Check sheet for the modelled part. Datum: model origin and axes. Units: mm. Round coordinates to 2 decimals unless told otherwise and drop trailing zeros. Write each loop counter-clockwise with the first axis right and the second up, starting at its lowest first coordinate (ties: lowest second). Pieces come first, ordered by that corner, then holes.
Item 1: Section check D-D, the plane y = 1.8. State how many separate pieces and enclosed holes the cut face has, plus the area to 3 significant figures.
Item 2: Material ranges on line 1 along X through (y, z) = (2.55, 39); line 2 along X through (y, z) = (0.75, 24.5); line 3 along X through (y, z) = (2.2, 43.5), recorded low to high.
Item 3: Section check A-A, the plane z = 49. Record the cut outline in (x, y).
Item 4: Section check C-C, the plane x = 16.25. Record the cut outline in (y, z), plus the area to 3 significant figures.
Item 5: Depth check by flat-ended pin: pin 1 (3.5 mm diameter, centred on x = -42.44, z = -24.5, fed in from -Y). Enter the tip coordinate at first touch or a pass-through.
Item 6: Section check B-B, the plane z = -36. Record the cut outline in (x, y), plus the area to 3 significant figures.
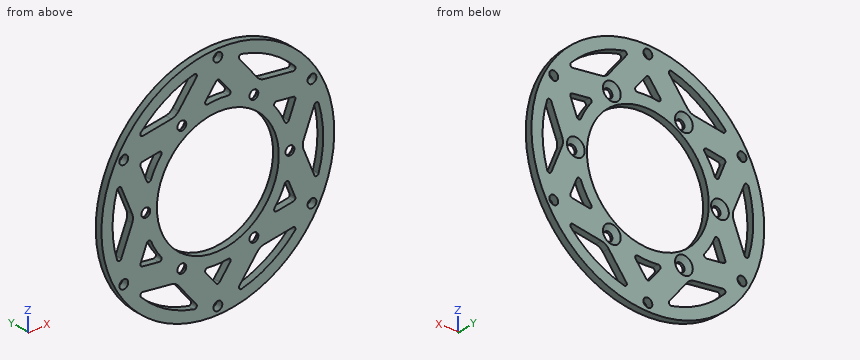
from build123d import *

# Parameters (mm, degrees)
SKETCH_1_R               = 52.5
SKETCH_1_R_2             = 2
SKETCH_1_R_3             = 27.5
EXTRUDE_1_DEPTH          = 3
HOLE_WIZARD_1_AT_2_COUNT = 2
HOLE_WIZARD_1_AT_2_PITCH = 32.5
HOLE_WIZARD_1_AT_3_COUNT = 2
HOLE_WIZARD_1_AT_3_PITCH = 56.291651246
HOLE_WIZARD_1_AT_4_COUNT = 2
HOLE_WIZARD_1_AT_4_PITCH = 65
HOLE_WIZARD_1_AT_5_COUNT = 2
HOLE_WIZARD_1_AT_5_PITCH = 56.291651246
HOLE_WIZARD_1_AT_6_COUNT = 2
HOLE_WIZARD_1_AT_6_PITCH = 32.5
CUT_EXTRUDE_1_DEPTH      = 10
FILLET_1_R               = 5
FILLET_2_R               = 1


with BuildPart() as part:
    # 草图1 → 凸台-拉伸1 (new body)
    with BuildSketch(Plane(origin=(0, 0, 0), x_dir=(1, 0, 0), z_dir=(0, 1, 0))):
        with Locations(Location((0, 0, 0), (0, 0, 270))):
            Circle(SKETCH_1_R)
        with Locations(Location((0, 49, 0), (0, 0, 270))):
            Circle(SKETCH_1_R_2, mode=Mode.SUBTRACT)
        with Locations(Location((-16.25, 28.145825623, 0), (0, 0, 270))):
            Circle(SKETCH_1_R_2, mode=Mode.SUBTRACT)
        with Locations(Location((42.435244785, 24.5, 0), (0, 0, 270))):
            Circle(SKETCH_1_R_2, mode=Mode.SUBTRACT)
        with Locations(Location((16.25, 28.145825623, 0), (0, 0, 270))):
            Circle(SKETCH_1_R_2, mode=Mode.SUBTRACT)
        with Locations(Location((42.435244785, -24.5, 0), (0, 0, 270))):
            Circle(SKETCH_1_R_2, mode=Mode.SUBTRACT)
        with Locations(Location((32.5, 0, 0), (0, 0, 270))):
            Circle(SKETCH_1_R_2, mode=Mode.SUBTRACT)
        with Locations(Location((0, -49, 0), (0, 0, 270))):
            Circle(SKETCH_1_R_2, mode=Mode.SUBTRACT)
        with Locations(Location((16.25, -28.145825623, 0), (0, 0, 270))):
            Circle(SKETCH_1_R_2, mode=Mode.SUBTRACT)
        with Locations(Location((-42.435244785, -24.5, 0), (0, 0, 270))):
            Circle(SKETCH_1_R_2, mode=Mode.SUBTRACT)
        with Locations(Location((-16.25, -28.145825623, 0), (0, 0, 270))):
            Circle(SKETCH_1_R_2, mode=Mode.SUBTRACT)
        with Locations(Location((-42.435244785, 24.5, 0), (0, 0, 270))):
            Circle(SKETCH_1_R_2, mode=Mode.SUBTRACT)
        with Locations(Location((-32.5, 0, 0), (0, 0, 270))):
            Circle(SKETCH_1_R_2, mode=Mode.SUBTRACT)
        with Locations(Location((0, 0, 0), (0, 0, 270))):
            Circle(SKETCH_1_R_3, mode=Mode.SUBTRACT)
    extrude(amount=EXTRUDE_1_DEPTH)

    # 草图3 → 孔1 (revolve, cut)
    with BuildSketch(Plane(origin=(-16.25, 3, -28.145825623), x_dir=(0, 0, 1), z_dir=(1, 0, 0))):
        Polygon((0, 0), (0, 3), (2, 3), (2, 2), (4, 0), align=None)
    hole_wizard_1 = revolve(axis=Axis((-16.25, 9.445314094, -28.145825623), (0, -1, 0)), mode=Mode.SUBTRACT)

    # 孔1 at 2: 孔1 ×2
    with Locations(*[(i * HOLE_WIZARD_1_AT_2_PITCH, 0, 0) for i in range(1, HOLE_WIZARD_1_AT_2_COUNT)]):
        add(hole_wizard_1, mode=Mode.SUBTRACT)

    # 孔1 at 3: 孔1 ×2
    with Locations(*[Vector(0.8660254037844387, 0, 0.5) * (i * HOLE_WIZARD_1_AT_3_PITCH) for i in range(1, HOLE_WIZARD_1_AT_3_COUNT)]):
        add(hole_wizard_1, mode=Mode.SUBTRACT)

    # 孔1 at 4: 孔1 ×2
    with Locations(*[Vector(0.5000000000000001, 0, 0.8660254037844386) * (i * HOLE_WIZARD_1_AT_4_PITCH) for i in range(1, HOLE_WIZARD_1_AT_4_COUNT)]):
        add(hole_wizard_1, mode=Mode.SUBTRACT)

    # 孔1 at 5: 孔1 ×2
    with Locations(*[(0, 0, i * HOLE_WIZARD_1_AT_5_PITCH) for i in range(1, HOLE_WIZARD_1_AT_5_COUNT)]):
        add(hole_wizard_1, mode=Mode.SUBTRACT)

    # 孔1 at 6: 孔1 ×2
    with Locations(*[Vector(-0.5000000000000003, 0, 0.8660254037844386) * (i * HOLE_WIZARD_1_AT_6_PITCH) for i in range(1, HOLE_WIZARD_1_AT_6_COUNT)]):
        add(hole_wizard_1, mode=Mode.SUBTRACT)

    # 草图5 → 切除-拉伸1 (cut)
    with BuildSketch(Plane(origin=(0, 3, 0), x_dir=(1, 0, 0), z_dir=(0, 1, 0))):
        with BuildLine():
            Line((-8.041886602, 46.814293329), (-18.947738206, 32.818445262))
            Line((-18.947738206, 32.818445262), (-36.521423982, 30.371624756))
            ThreePointArc((-36.521423982, 30.371624756), (-23.75, 41.13620668), (-8.041886602, 46.814293329))
        make_face()
        with BuildLine():
            Line((0, 40.865281716), (7.136483547, 31.706791111))
            ThreePointArc((7.136483547, 31.706791111), (0, 32.5), (-7.136483547, 31.706791111))
            Line((-7.136483547, 31.706791111), (0, 40.865281716))
        make_face()
        with BuildLine():
            Line((18.947738206, 32.818445262), (8.041886602, 46.814293329))
            ThreePointArc((8.041886602, 46.814293329), (23.75, 41.13620668), (36.521423982, 30.371624756))
            Line((36.521423982, 30.371624756), (18.947738206, 32.818445262))
        make_face()
        with BuildLine():
            Line((35.390372099, 20.432640858), (23.890644801, 22.033771601))
            ThreePointArc((23.890644801, 22.033771601), (28.145825623, 16.25), (31.027128348, 9.67301951))
            Line((31.027128348, 9.67301951), (35.390372099, 20.432640858))
        make_face()
        with BuildLine():
            Line((37.895476413, 0), (44.563310584, 16.442668573))
            ThreePointArc((44.563310584, 16.442668573), (47.5, 0), (44.563310584, -16.442668573))
            Line((44.563310584, -16.442668573), (37.895476413, 0))
        make_face()
        with BuildLine():
            Line((35.390372099, -20.432640858), (31.027128348, -9.67301951))
            ThreePointArc((31.027128348, -9.67301951), (28.145825623, -16.25), (23.890644801, -22.033771601))
            Line((23.890644801, -22.033771601), (35.390372099, -20.432640858))
        make_face()
        with BuildLine():
            Line((18.947738206, -32.818445262), (36.521423982, -30.371624756))
            ThreePointArc((36.521423982, -30.371624756), (23.75, -41.13620668), (8.041886602, -46.814293329))
            Line((8.041886602, -46.814293329), (18.947738206, -32.818445262))
        make_face()
        with BuildLine():
            Line((0, -40.865281716), (7.136483547, -31.706791111))
            ThreePointArc((7.136483547, -31.706791111), (0, -32.5), (-7.136483547, -31.706791111))
            Line((-7.136483547, -31.706791111), (0, -40.865281716))
        make_face()
        with BuildLine():
            Line((-18.947738206, -32.818445262), (-8.041886602, -46.814293329))
            ThreePointArc((-8.041886602, -46.814293329), (-23.75, -41.13620668), (-36.521423982, -30.371624756))
            Line((-36.521423982, -30.371624756), (-18.947738206, -32.818445262))
        make_face()
        with BuildLine():
            Line((-35.390372099, -20.432640858), (-23.890644801, -22.033771601))
            ThreePointArc((-23.890644801, -22.033771601), (-28.145825623, -16.25), (-31.027128348, -9.67301951))
            Line((-31.027128348, -9.67301951), (-35.390372099, -20.432640858))
        make_face()
        with BuildLine():
            Line((-37.895476413, 0), (-44.563310584, -16.442668573))
            ThreePointArc((-44.563310584, -16.442668573), (-47.5, 0), (-44.563310584, 16.442668573))
            Line((-44.563310584, 16.442668573), (-37.895476413, 0))
        make_face()
        with BuildLine():
            Line((-35.390372099, 20.432640858), (-31.027128348, 9.67301951))
            ThreePointArc((-31.027128348, 9.67301951), (-28.145825623, 16.25), (-23.890644801, 22.033771601))
            Line((-23.890644801, 22.033771601), (-35.390372099, 20.432640858))
        make_face()
    extrude(amount=-CUT_EXTRUDE_1_DEPTH, mode=Mode.SUBTRACT)

    # 圆角1
    fillet_1_edges = [part.edges().sort_by_distance(p)[0] for p in [
        (-18.947738206, 1.5, 32.818445262),
        (18.947738206, 1.5, 32.818445262),
        (37.895476413, 1.5, 0),
        (18.947738206, 1.5, -32.818445262),
        (-37.895476413, 1.5, 0),
        (-18.947738206, 1.5, -32.818445262),
    ]]
    fillet(fillet_1_edges, radius=FILLET_1_R)

    # 圆角2
    fillet_2_edges = [part.edges().sort_by_distance(p)[0] for p in [
        (-8.041886602, 1.5, 46.814293329),
        (-36.521423982, 1.5, 30.371624756),
        (0, 1.5, 40.865281716),
        (-7.136483547, 1.5, 31.706791111),
        (7.136483547, 1.5, 31.706791111),
        (36.521423982, 1.5, 30.371624756),
        (8.041886602, 1.5, 46.814293329),
        (35.390372099, 1.5, 20.432640858),
        (23.890644801, 1.5, 22.033771601),
        (31.027128348, 1.5, 9.67301951),
        (44.563310584, 1.5, -16.442668573),
        (44.563310584, 1.5, 16.442668573),
        (35.390372099, 1.5, -20.432640858),
        (31.027128348, 1.5, -9.67301951),
        (23.890644801, 1.5, -22.033771601),
        (8.041886602, 1.5, -46.814293329),
        (36.521423982, 1.5, -30.371624756),
        (-7.136483547, 1.5, -31.706791111),
        (0, 1.5, -40.865281716),
        (7.136483547, 1.5, -31.706791111),
        (-35.390372099, 1.5, -20.432640858),
        (-23.890644801, 1.5, -22.033771601),
        (-31.027128348, 1.5, -9.67301951),
        (-44.563310584, 1.5, 16.442668573),
        (-44.563310584, 1.5, -16.442668573),
        (-35.390372099, 1.5, 20.432640858),
        (-31.027128348, 1.5, 9.67301951),
        (-23.890644801, 1.5, 22.033771601),
        (-36.521423982, 1.5, -30.371624756),
        (-8.041886602, 1.5, -46.814293329),
    ]]
    fillet(fillet_2_edges, radius=FILLET_2_R)


solid = part.part
Values found:
1. separate pieces: 1
1. enclosed holes: 25
1. area: 4,710 mm2
2. line 1: x = -35.15 to -27.12, -14.13 to -1.45, 1.45 to 14.13, 27.12 to 35.15
2. line 2: x = -46.43 to -44.44, -40.44 to -12.49, 12.49 to 40.44, 44.44 to 46.43
2. line 3: x = -29.39 to -19.08, -10.62 to 10.62, 19.08 to 29.39
3. outline: (-18.85, 0) - (-2, 0) - (-2, 3) - (-18.85, 3) - close; (2, 0) - (18.85, 0) - (18.85, 3) - (2, 3) - close
4. outline: (0, -49.92) - (3, -49.92) - (3, -44.63) - (0, -44.63) - close; (0, -36.28) - (3, -36.28) - (3, -32.15) - (1, -30.15) - (0, -30.15) - close; (0, -26.15) - (1, -26.15) - (3, -24.15) - (3, -22.19) - (0, -22.19) - close; (0, 22.19) - (3, 22.19) - (3, 24.15) - (1, 26.15) - (0, 26.15) - close; (0, 30.15) - (1, 30.15) - (3, 32.15) - (3, 36.28) - (0, 36.28) - close; (0, 44.63) - (3, 44.63) - (3, 49.92) - (0, 49.92) - close
4. area: 84.3 mm2
5. pin 1: passes through
6. outline: (-38.21, 0) - (-30.99, 0) - (-30.99, 3) - (-38.21, 3) - close; (-16.47, 0) - (-3.79, 0) - (-3.79, 3) - (-16.47, 3) - close; (3.79, 0) - (16.47, 0) - (16.47, 3) - (3.79, 3) - close; (30.99, 0) - (38.21, 0) - (38.21, 3) - (30.99, 3) - close
6. area: 119 mm2
